Read the model definition and answer for the solid it produces. Units are mm, in the model's axes. Face numbers are marked on the shaded views. A direction names the side the tool comes from. Round coordinates to 2 decimals unless told otherwise and drop trailing zeros. Loops run counter-clockwise (first coordinate to the right, second up) from the corner with the lowest first, then second, coordinate; pieces in that order, holes last. Notation, with made-up numbers: M 27,19.5 L 41,19.5 A17 ccw 41,42.5 Z; hole C 25.25,-16 d2. An arc over 180 degrees is marked long. Write each question's results on one line, items separated by ' | '.
from build123d import *

# Parameters (mm, degrees)
SKETCH1_R                 = 22.5
BOSS_EXTRUDE1_DEPTH       = 20
CUT_EXTRUDE1_REACH        = 22
SKETCH3_R                 = 9.5
F_3_0MM_DOWEL_HOLE1_D     = 3
F_3_0MM_DOWEL_HOLE1_DEPTH = 22
F_3_0MM_DOWEL_HOLE1_TIP   = 0.901291
BOSS_EXTRUDE3_DEPTH       = 10


with BuildPart() as part:
    # Sketch1 → Boss-Extrude1 (new body)
    with BuildSketch(Plane.XY):
        Circle(SKETCH1_R)
    extrude(amount=BOSS_EXTRUDE1_DEPTH)

    # Sketch3 → Cut-Extrude1 (cut, up to next)
    with BuildSketch(Plane.XY.offset(20), mode=Mode.PRIVATE) as cut_extrude1_sk1:
        Circle(SKETCH3_R)
    cut_extrude1_tool1 = extrude(cut_extrude1_sk1.sketch, amount=-CUT_EXTRUDE1_REACH, mode=Mode.PRIVATE) & part.part
    add(cut_extrude1_tool1.solids().sort_by_distance((0, 0, 20))[0], mode=Mode.SUBTRACT)

    # Ø3.0mm Dowel Hole1
    with Locations(Plane(origin=(0.332625, 22.497541, 9.950984), x_dir=(0.999891, -0.014783, 0), z_dir=(0.014783, 0.999891, 0))):
        with Locations((0, 0)):
            Hole(F_3_0MM_DOWEL_HOLE1_D / 2, depth=F_3_0MM_DOWEL_HOLE1_DEPTH)
            with Locations((0, 0, -(F_3_0MM_DOWEL_HOLE1_DEPTH + F_3_0MM_DOWEL_HOLE1_TIP / 2))):  # 118° drill point
                Cone(0, F_3_0MM_DOWEL_HOLE1_D / 2, F_3_0MM_DOWEL_HOLE1_TIP, mode=Mode.SUBTRACT)

    # Sketch6 → Boss-Extrude3 (add)
    with BuildSketch(Plane.XY.offset(20)):
        with BuildLine():
            Line((-17.498377, 14.144144), (-10.881805, 10.324065))
            ThreePointArc((-10.881805, 10.324065), (-7.5, 12.990381), (-3.5, 14.585952))
            Line((-3.5, 14.585952), (-3.5, 22.226111))
            ThreePointArc((-3.5, 22.226111), (-11.25, 19.485572), (-17.498377, 14.144144))
        make_face()
        with BuildLine():
            Line((14.381805, 4.261887), (20.998377, 8.081966))
            ThreePointArc((20.998377, 8.081966), (22.5, 0), (20.998377, -8.081966))
            Line((20.998377, -8.081966), (14.381805, -4.261887))
            ThreePointArc((14.381805, -4.261887), (15, 0), (14.381805, 4.261887))
        make_face()
        with BuildLine():
            Line((-3.5, -14.585952), (-3.5, -22.226111))
            ThreePointArc((-3.5, -22.226111), (-11.25, -19.485572), (-17.498377, -14.144144))
            Line((-17.498377, -14.144144), (-10.881805, -10.324065))
            ThreePointArc((-10.881805, -10.324065), (-7.5, -12.990381), (-3.5, -14.585952))
        make_face()
    extrude(amount=BOSS_EXTRUDE3_DEPTH)


solid = part.part
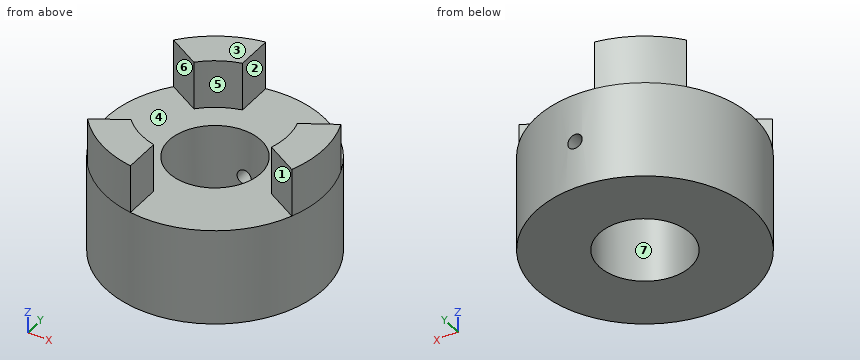
Item 1: Flat-ended cylindrical pins translate along their axes: pin 1 (5 mm diameter, centred on y = -17.5, z = 11.5, fed in from +X); pin 2 (6 mm diameter, centred on x = 7.5, z = 6.5, fed in from +Y); pin 3 (3 mm diameter, centred on y = -3.5, z = 24, fed in from -X); pin 4 (15 mm diameter, centred on x = 0, y = 0, fed in from -Z). Find the tip coordinate at first contact, or state that the pin passes through.
Outcome:
pin 1: stops at x = 16.77 | pin 2: stops at y = 22.05 | pin 3: stops at x = 14.38 | pin 4: passes through
Item 2: The part is cut by section D-D (x = -14.5). Determine the outline of the cut face in (y, z), plus the area to 3 significant figures.
Outcome:
outline: M -17.2,0 L 17.2,0 L 17.2,30 L 12.41,30 L 12.41,20 L -12.41,20 L -12.41,30 L -17.2,30 Z | area: 784 mm2
Item 3: The mould has two halves that part along X. Classify the marked faces 4, 5, 6 and 7: pulls with the +X half, pulls with the -X half, needs draft (parallel to the pull), parting line crosses it, or undercut.
Outcome:
face 4: needs draft | face 5: pulls with the +X half | face 6: pulls with the -X half | face 7: undercut
Item 4: For the marked faces 1, 2 and 3, determine the directions among +Z, -Z, +X, -X, +Y, -Y from which every point of the face is accessible in a straight line to the end or side of a thin tool.
Outcome:
face 1: +Z, -X, -Y | face 2: +Z, +X, +Y, -Y | face 3: +Z, +X, -X, +Y, -Y
Item 5: Straight lines are drawn through the part: line 1 (Y direction, x = 0, z = 5.75); line 2 (X direction, y = -17.5, z = 6); line 3 (Z direction, x = 0, y = -16). For each, find the intervals that lie inside material, in ascending order.
Outcome:
line 1: y = -22.5 to -9.5, 9.5 to 22.5 | line 2: x = -14.14 to 14.14 | line 3: z = 0 to 20
Item 6: The part is cut by section A-A (y = 0). Determine the outline of the cut face in (x, z).
Outcome:
outline: M -22.5,0 L -9.5,0 L -9.5,20 L -22.5,20 Z; M 9.5,0 L 22.5,0 L 22.5,30 L 15,30 L 15,20 L 9.5,20 Z
Item 7: The part is cut by section B-B (z = 22.5). Determine the outline of the cut face in (x, y), plus the area to 3 significant figures.
Outcome:
outline: M -17.5,-14.14 A22.5 ccw -3.5,-22.23 L -3.5,-14.59 A15 cw -10.88,-10.32 Z; M -17.5,14.14 L -10.88,10.32 A15 cw -3.5,14.59 L -3.5,22.23 A22.5 ccw Z; M 14.38,-4.26 L 21,-8.08 A22.5 ccw 21,8.08 L 14.38,4.26 A15 cw Z | area: 283 mm2
Item 8: The part is cut by section C-C (y = -18). Determine the outline of the cut face in (x, z).
Outcome:
outline: M -13.5,0 L 13.5,0 L 13.5,20 L -3.5,20 L -3.5,30 L -13.5,30 Z
